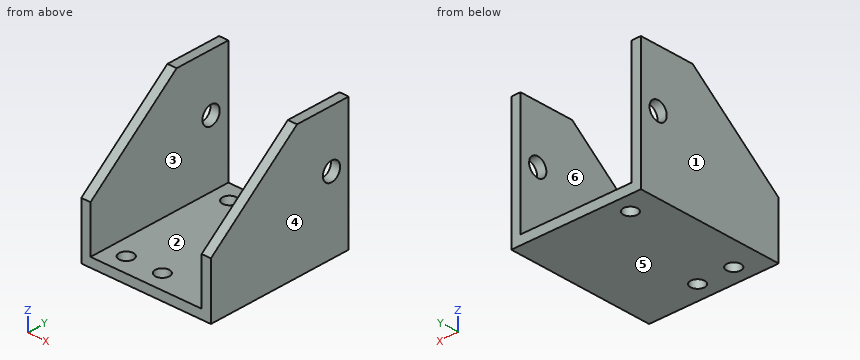
Autodesk Inventor part; units mm, degrees
ref_plane "YZ Plane" through (0, 0, 0) normal (1, 0, 0) x (0, 1, 0)
ref_plane "XZ Plane" through (0, 0, 0) normal (0, 1, 0) x (-1, 0, 0)
ref_plane "XY Plane" through (0, 0, 0) normal (0, 0, 1) x (1, 0, 0)
sketch "Sketch1" plane through (0, 0, 0) normal (0, 1, 0) x (-1, 0, 0)
  line L0 (0, 0) -> (44.45, 0)
  line L1 (44.45, 0) -> (44.45, -44.45)
  line L2 (44.45, -44.45) -> (0, -44.45)
  line L3 (0, -44.45) -> (0, 0)
  line L4 (41.275, -41.275) -> (41.275, -3.175)
  line L5 (41.275, -3.175) -> (3.175, -3.175)
  line L6 (3.175, -3.175) -> (3.175, -41.275)
  line L7 (3.175, -41.275) -> (41.275, -41.275)
  line L8 (41.275, -3.175) -> (41.275, 0)
  line L9 (3.175, -3.175) -> (3.175, 0)
  dimension "d0" = 3.175
  dimension "d1" = 44.45
extrude "Extrusion1" add sketch "Sketch1" along normal blind 50.8 contours L0 L9 L6 L7 L4 L8 L1 L2 L3
sketch "Sketch2" plane through (0, 0, 0) normal (1, 0, 0) x (0, 0, -1)
  line L0 (0, 50.8) -> (44.45, 50.8)
  line L1 (0, 0) -> (0, 50.8)
  line L2 (44.45, 0) -> (44.45, 50.8)
  point P0 (19.05, 44.45)
  dimension "d11" = 6.35
  dimension "d13" = 25.4
hole "Hole1" at (0, 44.45, -19.05) direction (-1, 0, 0) diameter 6.35 end through all
sketch "Sketch3" plane through (0, 0, -44.45) normal (0, 0, -1) x (-1, 0, 0)
  line L0 (16.2052, 86.1658) -> (16.2052, -32.4239) construction
  line L1 (0, 0) -> (0, 50.8) construction
  line L2 (44.45, 0) -> (44.45, 50.8) construction
  line L3 (0, 50.8) -> (44.45, 50.8) construction
  line L4 (0, 0) -> (44.45, 0)
  point P0 (34.925, 44.45)
  point P1 (34.925, 6.35)
  point P2 (22.5552, 6.35)
  point P3 (22.5552, 44.45)
  dimension "d14" = 16.2052
  dimension "d17" = 6.35
  dimension "d18" = 6.35
  dimension "d19" = 6.35
  dimension "d30" = 6.35
  dimension "d31" = 9.525
  dimension "d32" = 9.525
  dimension "d33" = 6.35
  dimension "d34" = 6.35
hole "Hole2" at (-34.925, 44.45, -44.45) at (-34.925, 6.35, -44.45) at (-22.5552, 6.35, -44.45) direction (0, 0, 1) diameter 4.826 end through all
sketch "Sketch4" plane through (-44.45, 0, -44.45) normal (-1, 0, 0) x (0, 0, 1)
  line L0 (19.05, 0) -> (44.45, 31.75)
  circle A0 centre (25.4, 44.45) radius 3.175
  line L1 (0, 0) -> (44.45, 0)
  line L2 (44.45, 0) -> (44.45, 50.8)
  line L3 (0, 50.8) -> (44.45, 50.8)
  line L4 (0, 0) -> (0, 50.8)
  point P0 (44.45, 0)
  dimension "d35" = 19.05
  dimension "d36" = 25.4
extrude "Extrusion2" cut sketch "Sketch4" against normal blind 152.4 contours L0 L2 L1
properties part number "CAR_016_TensionerMount" material "Aluminum 6061"
Work out the finished part from the listing and answer in its coordinate system (mm). Face numbers are marked on the shaded views. A direction names the side the tool comes from. Round coordinates to 2 decimals unless told otherwise and drop trailing zeros. Loops run counter-clockwise (first coordinate to the right, second up) from the corner with the lowest first, then second, coordinate; pieces in that order, holes last.
(1) The part is cut by section D-D, the plane z = -19.05. Give the number of separate pieces and of enclosed holes in the cut face, and give its area (3 significant figures).
Computed values:
separate pieces: 4
enclosed holes: 0
area: 232 mm2
(2) The part is cut by section C-C, the plane y = 6.35. Give the vertices of the cut face in (x, z) (3 decimals).
Computed values:
outline: (-44.45, -44.45) - (-37.338, -44.45) - (-37.338, -41.275) - (-41.275, -41.275) - (-41.275, -20.32) - (-44.45, -20.32) - close; (-32.512, -44.45) - (-24.968, -44.45) - (-24.968, -41.275) - (-32.512, -41.275) - close; (-20.142, -44.45) - (0, -44.45) - (0, -20.32) - (-3.175, -20.32) - (-3.175, -41.275) - (-20.142, -41.275) - close
(3) For the marked faces 1 and 2, determine the directions among +Z, -Z, +X, -X, +Y, -Y from which every point of the face is accessible in a straight line to the end or side of a thin tool.
Computed values:
face 1: +Z, -Z, -X, +Y, -Y
face 2: +Z, +Y, -Y
(4) The mould has two halves that part along X. Classify the marked faces 3, 4, 5 and 6: pulls with the +X half, pulls with the -X half, needs draft (parallel to the pull), parting line crosses it, or undercut.
Computed values:
face 3: undercut
face 4: pulls with the +X half
face 5: needs draft
face 6: undercut
(5) The part is cut by section A-A, the plane y = 44.45. Give the vertices of the cut face in (x, z) (3 decimals), and give its area (3 significant figures).
Computed values:
outline: (-44.45, -44.45) - (-37.338, -44.45) - (-37.338, -41.275) - (-41.275, -41.275) - (-41.275, -22.225) - (-44.45, -22.225) - close; (-44.45, -15.875) - (-41.275, -15.875) - (-41.275, 0) - (-44.45, 0) - close; (-32.512, -44.45) - (0, -44.45) - (0, -22.225) - (-3.175, -22.225) - (-3.175, -41.275) - (-32.512, -41.275) - close; (-3.175, -15.875) - (0, -15.875) - (0, 0) - (-3.175, 0) - close
area: 348 mm2
(6) Each of these flat-tipped pins is pushed along its axis until it touches: P1, Ø7.5, axis at y = 44.45, z = -19.05, coming from the +X side; P2, Ø4, axis at x = -34.5, z = -39, coming from the -Y side; P3, Ø6.5, axis at x = -22.56, y = 6.35, coming from the +Z side (3 decimals). Where does it stop, or does it pass through?
Computed values:
P1: stops at x = 0
P2: passes through
P3: stops at z = -41.275
(7) The part is cut by section B-B, the plane z = -34.5. Give the vertices of the cut face in (x, y) (3 decimals), and give its area (3 significant figures).
Computed values:
outline: (-44.45, 0) - (-41.275, 0) - (-41.275, 50.8) - (-44.45, 50.8) - close; (-3.175, 0) - (0, 0) - (0, 50.8) - (-3.175, 50.8) - close
area: 323 mm2
(8) Find the intervals of material crossed by L1, parallel to X at y = 6.35, z = -43.25; L2, parallel to X at y = 44.45, z = -42.4; L3, parallel to Z at x = -43.4, y = 44.45 (3 decimals), in increasing order.
Computed values:
L1: x = -44.45 to -37.34, -32.51 to -24.97, -20.14 to 0
L2: x = -44.45 to -37.34, -32.51 to 0
L3: z = -44.45 to -22.225, -15.875 to 0
